Here's how the part is built. I have some questions about the finished solid (model axes, mm). A direction names the side the tool comes from. Coordinates: 2 decimals unless noted, no trailing zeros. Write each loop counter-clockwise with the first axis right and the second up, starting at its lowest first coordinate (ties: lowest second). Pieces come first, ordered by that corner, then holes. Notation, with made-up numbers: (69, 80.5) - (80, 80.5) arc R16 ccw to (80, 89.5) - close; hole circle Ø5 at (0, 20). An arc over 180 degrees is marked (long way). Answer in a Markdown table with one row per item. Add a question column.
Item 1: If I drill on probe 1 along Y at (x, z) = (0, 0.3); probe 2 along Y at (x, z) = (0, 116.5); probe 3 along Y at (x, z) = (-1.5, 108.5), over which ranges is the centre line in solid material (lowest first)? Write a range as from..to.
Item 2: I'm going to push flat-ended pins straight in: pin 1 (2.5 mm diameter, centred on y = -2, z = 131.5, fed in from +X); pin 2 (2.5 mm diameter, centred on y = 2, z = 129, fed in from -X); pin 3 (10.5 mm diameter, centred on x = 0, y = 0, fed in from +Z). Where does each tip first touch, or does it pass through?
Item 3: Imagine slicing it at A-A (z = 55.5). Please give me the cut outline in (x, y).
Item 4: Imagine slicing it at C-C (y = 42.5). Please give me the cut outline in (x, z).
Item 5: Imagine slicing it at B-B (x = -45). Please give me the cut outline in (y, z), plus the area to 3 significant figures.
Item 6: Which directions (+Z, -Z, +X, -X, +Y, -Y) give clear straight access to the entire face, cutting with the end or side of a thin tool? Please do faces 1 (the face through (17.983, -0.791, 68.597)), 2 (the face through (-16, 0, 131)), 3 (the face through (16, 0, 131)), 4 (the face through (-16, -7, 1)).
Item 7: We'd pull the mould along Y, two halves only. Please class faces 5 (the face through (-9.139, 14.334, 0.493)), 6 (the face through (-13, -13, 5)), 7 (the face through (-8.071, 61.472, 2.535)): +Y half, -Y half, draft (parallel to the pull), parting line (faces both ways), or undercut.
from build123d import *

# Parameters (mm, degrees)
SKETCH1_R                   = 18
BASE_EXTRUDE_DEPTH          = 5
SKETCH6_R                   = 18
SKETCH6_R_2                 = 17
CUT_EXTRUDE1_DEPTH          = 1
SKETCH7_R                   = 18
BOSS_EXTRUDE1_DEPTH         = 130
CHAMFER1_SIZE               = 1
SKETCH2_W                   = 10
SKETCH2_H                   = 30
WRENCHFLATS_DEPTH           = 11
WRENCHFLATSCHAMFER_SIZE     = 2
SKETCH3_R                   = 5
INTERNALTHREAD_DEPTH        = 30
INTERNALTHREADCHAMFER_SIZE  = 1.2
PISTON_OUTLINE_W            = 44
PISTON_OUTLINE_H            = 5
F_3_4_16_TAPPED_HOLE1_D     = 17.4625
F_3_4_16_TAPPED_HOLE1_DEPTH = 34.76
F_3_4_16_TAPPED_HOLE1_TIP   = 5.24626428
CHAMFER2_SIZE               = 1


# Read off the part's stored shape, not the designer's step: Piston
with BuildPart() as part:
    # Sketch1 → Base-Extrude (new body)
    with BuildSketch(Plane.XY):
        Circle(SKETCH1_R)
    extrude(amount=BASE_EXTRUDE_DEPTH)

    # Sketch6 → Cut-Extrude1 (cut)
    with BuildSketch(Plane(origin=(0, 0, 0), x_dir=(-1, 0, 0), z_dir=(0, 0, -1))):
        Circle(SKETCH6_R)
        Circle(SKETCH6_R_2, mode=Mode.SUBTRACT)
    extrude(amount=-CUT_EXTRUDE1_DEPTH, mode=Mode.SUBTRACT)

    # Sketch7 → Boss-Extrude1 (add)
    with BuildSketch(Plane.XY.offset(5)):
        with Locations(Location((0, 0, 0), (0, 0, 180))):
            Circle(SKETCH7_R)
    extrude(amount=BOSS_EXTRUDE1_DEPTH)

    # Chamfer1
    chamfer1_edges = [part.edges().sort_by_distance(p)[0] for p in [
        (18, 0, 135),
    ]]
    chamfer(chamfer1_edges, length=CHAMFER1_SIZE)

    # Sketch2 → WrenchFlats (cut)
    with BuildSketch(Plane.XY.offset(135)):
        with Locations((21, 0)):
            Rectangle(SKETCH2_W, SKETCH2_H)
        with Locations((-21, 0)):
            Rectangle(SKETCH2_W, SKETCH2_H)
    extrude(amount=-WRENCHFLATS_DEPTH, mode=Mode.SUBTRACT)

    # WrenchFlatsChamfer
    wrenchflatschamfer_edges = [part.edges().sort_by_distance(p)[0] for p in [
        (16, 0, 124),
        (-16, 0, 124),
    ]]
    chamfer(wrenchflatschamfer_edges, length=WRENCHFLATSCHAMFER_SIZE - 0.0001)  # a hair under: the kernel refuses the full size

    # Sketch3 → InternalThread (cut)
    with BuildSketch(Plane.XY.offset(135)):
        Circle(SKETCH3_R)
    extrude(amount=-INTERNALTHREAD_DEPTH, mode=Mode.SUBTRACT)

    # InternalThreadChamfer
    internalthreadchamfer_edges = [part.edges().sort_by_distance(p)[0] for p in [
        (-5, 0, 135),
    ]]
    chamfer(internalthreadchamfer_edges, length=INTERNALTHREADCHAMFER_SIZE)

    # Piston outline → Piston (revolve)
    with BuildSketch(Plane.XZ):
        with Locations((40, 2.5)):
            Rectangle(PISTON_OUTLINE_W, PISTON_OUTLINE_H)
    revolve(axis=Axis((0, 0, 0), (0, 0, 1)))

    # 3/4-16 Tapped Hole1
    with Locations(Plane.XY.offset(135)):
        with Locations((0, 0)):
            Hole(F_3_4_16_TAPPED_HOLE1_D / 2, depth=F_3_4_16_TAPPED_HOLE1_DEPTH)
            with Locations((0, 0, -(F_3_4_16_TAPPED_HOLE1_DEPTH + F_3_4_16_TAPPED_HOLE1_TIP / 2))):  # 118° drill point
                Cone(0, F_3_4_16_TAPPED_HOLE1_D / 2, F_3_4_16_TAPPED_HOLE1_TIP, mode=Mode.SUBTRACT)

    # Chamfer2
    chamfer2_edges = [part.edges().sort_by_distance(p)[0] for p in [
        (8.73125, 0, 135),
    ]]
    chamfer(chamfer2_edges, length=CHAMFER2_SIZE)


solid = part.part
Here are the results:
| question | item | result |
|---|---|---|
| 1 | probe 1 | y = -62..-18, -17..17, 18..62 |
| 1 | probe 2 | y = -18..-8.73, 8.73..18 |
| 1 | probe 3 | y = -17.94..-8.6, 8.6..17.94 |
| 2 | pin 1 | stops at x = 16 |
| 2 | pin 2 | stops at x = -16 |
| 2 | pin 3 | stops at z = 98.15 |
| 3 | outline | circle Ø36 at (0, 0) |
| 4 | outline | (-45.14, 0) - (45.14, 0) - (45.14, 5) - (-45.14, 5) - close |
| 5 | outline | (-42.65, 0) - (42.65, 0) - (42.65, 5) - (-42.65, 5) - close |
| 5 | area | 426 mm2 |
| 6 | face 1 | +Z |
| 6 | face 2 | +Z, -X, +Y, -Y |
| 6 | face 3 | +Z, +X, +Y, -Y |
| 6 | face 4 | -Z |
| 7 | face 5 | undercut |
| 7 | face 6 | draft |
| 7 | face 7 | parting line |
